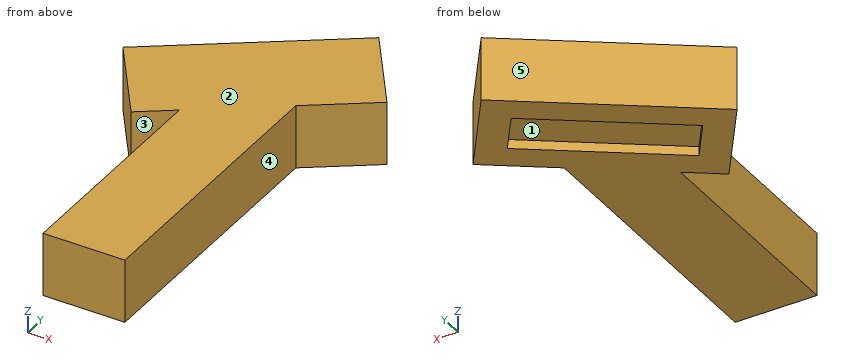
from build123d import *

# Parameters (mm, degrees)
SALIENTE_EXTRUIR1_DEPTH = 38
CORTAR_EXTRUIR4_START   = -38
CORTAR_EXTRUIR4_DEPTH   = 11


with BuildPart() as part:
    # Croquis1 → Saliente-Extruir1 (new, symmetric)
    with BuildSketch(Plane.XY):
        Polygon((-1.079549163, -361), (61.920450837, -361), (61.920450837, -21.313279486), (138.671836045, 32.428619004), (68.69551081, 132.365168408), (-146.741476838, -18.485434353), (-76.765151603, -118.421983756), (-36.079549163, -89.933618231), (-36.079549163, -361), align=None)
    extrude(amount=SALIENTE_EXTRUIR1_DEPTH, both=True)

    # Croquis2 → Cortar-Extruir4 (cut, symmetric)
    with BuildSketch(Plane.XY.offset(CORTAR_EXTRUIR4_START)):
        Polygon((-101.068225195, -26.179853393), (-68.374368323, -72.871519917), (92.998584402, 40.123038044), (60.30472753, 86.814704569), align=None)
    extrude(amount=CORTAR_EXTRUIR4_DEPTH, both=True, mode=Mode.SUBTRACT)


solid = part.part
Could you check a few things on this model? Use its own coordinates, in mm. Face numbers are marked on the shaded views. A direction names the side the tool comes from. Round coordinates to 2 decimals unless told otherwise and drop trailing zeros. Order: outer loops, then holes, each group sorted by start corner. A loop starts at its lowest first (then second) coordinate and runs counter-clockwise, first axis right, second up.
(1) Imagine slicing it at B-B (y = -112). Write out the boundary of the cut face in (x, z), plus the area to 3 significant figures.
Response values:
outline: (-81.26, -38) - (-67.59, -38) - (-67.59, 38) - (-81.26, 38) - close; (-36.08, -38) - (61.92, -38) - (61.92, 38) - (-36.08, 38) - close
area: 8,490 mm2
(2) Which directions (+Z, -Z, +X, -X, +Y, -Y) give clear straight access to the entire face, cutting with the end or side of a thin tool? Please do the marked faces 1 and 2.
Response values:
face 1: -Z
face 2: +Z, +X, -X, +Y, -Y
(3) Imagine slicing it at D-D (y = -198.5). Write out the boundary of the cut face in (x, z).
Response values:
outline: (-36.08, -38) - (61.92, -38) - (61.92, 38) - (-36.08, 38) - close
(4) Imagine slicing it at A-A (z = 30). Write out the boundary of the cut face in (x, y), plus the area to 3 significant figures.
Response values:
outline: (-146.74, -18.49) - (-76.77, -118.42) - (-36.08, -89.93) - (-36.08, -361) - (61.92, -361) - (61.92, -21.31) - (138.67, 32.43) - (68.7, 132.37) - close
area: 62,000 mm2
(5) Imagine slicing it at C-C (x = 0.5). Write out the boundary of the cut face in (y, z), plus the area to 3 significant figures.
Response values:
outline: (-361, -38) - (-24.65, -38) - (-24.65, -27) - (44.94, -27) - (44.94, -38) - (84.61, -38) - (84.61, 38) - (-361, 38) - close
area: 33,100 mm2
(6) Please list where these lines run through material, in increasing order: line 1 along Z through (x, y) = (-18, -2); line 2 along X through (y, z) = (-201, 19); line 3 along X through (y, z) = (-54, 35).
Response values:
line 1: z = -27 to 38
line 2: x = -36.08 to 61.92
line 3: x = -121.87 to 61.92
(7) I'm going to push flat-ended pins straight in: pin 1 (5 mm diameter, centred on x = -92.5, z = -11.5, fed in from +Y); pin 2 (10 mm diameter, centred on y = -76.5, z = -25.5, fed in from +X); pin 3 (1 mm diameter, centred on x = 93, z = -24, fed in from -Y); pin 4 (4 mm diameter, centred on x = -47, y = -100.5, fed in from +Z). Where does each tip first touch, or does it pass through?
Response values:
pin 1: stops at y = 21.25
pin 2: stops at x = 61.92
pin 3: stops at y = 0.1
pin 4: passes through
(8) If we mould it in two halves opening along X, with no side actions, what happens to the marked faces 3, 4 and 5? For each: released by +X, released by -X, zero draft, split by the parting line, or undercut.
Response values:
face 3: undercut
face 4: released by +X
face 5: released by -X
